Could you check a few things on this model? Use its own coordinates, in mm. Face numbers are marked on the shaded views. Round coordinates to 2 decimals unless told otherwise and drop trailing zeros. Write each loop counter-clockwise with the first axis right and the second up, starting at its lowest first coordinate (ties: lowest second). Pieces come first, ordered by that corner, then holes. Notation, with made-up numbers: (58.5, 80.25) -> (93.5, 80.25) arc R9 ccw to (93.5, 85.25) -> close; hole circle Ø8 at (6.25, 62.25). An arc over 180 degrees is marked (long way). Answer in a Markdown table with one row per item.
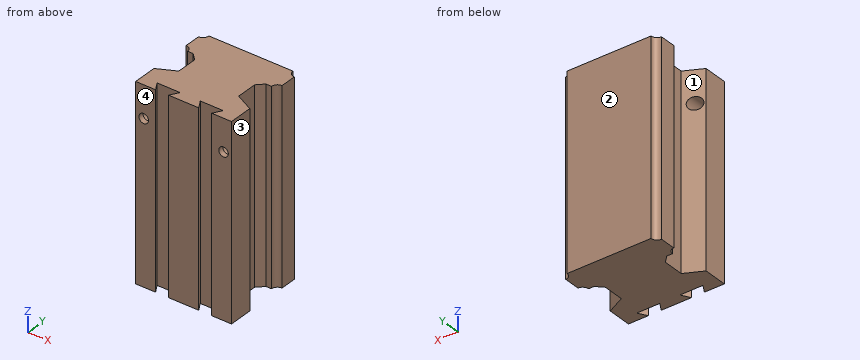
from build123d import *

# Parameters (mm, degrees)
BOSS_EXTRU_1_DEPTH        = 38.1
CONG_1_R                  = 2.38125
CHANFREIN1_SIZE           = 10.16
CHANFREIN1_SIZE_2         = 5.08
CHANFREIN2_SIZE           = 10.16
CHANFREIN2_SIZE_2         = 5.08
CHANFREIN3_SIZE           = 2.54
EMPREINTE1_START          = -38.1
EMPREINTE1_DEPTH          = 76.2
D_PLACER_START            = -38.1
D_PLACER_LA_FACE1_DEPTH   = 76.2
ESQUISSE4_W               = 1.89865
ESQUISSE4_H               = 21.2725
D_GAGEMENT_61_AT_2_COUNT  = 2
D_GAGEMENT_61_AT_2_PITCH  = 31.75
D_GAGEMENT_101_AT_2_COUNT = 2
D_GAGEMENT_101_AT_2_PITCH = 31.75


# Read off the part's stored shape, not the designer's step: Empreinte1, Déplacer la face1
# Some blends are built 0.0001 mm under size
with BuildPart() as part:
    # Esquisse2 → Boss.-Extru.1 (new, symmetric)
    with BuildSketch(Plane.XY):
        Polygon((-19.05, -15.875), (19.05, -15.875), (19.05, -7.9375), (11.90625, -7.9375), (11.90625, 7.9375), (16.66875, 7.9375), (16.66875, 10.31875), (19.05, 10.31875), (19.05, 16.66875), (16.66875, 16.66875), (16.66875, 19.05), (-16.66875, 19.05), (-16.66875, 16.66875), (-19.05, 16.66875), (-19.05, 10.31875), (-16.66875, 10.31875), (-16.66875, 7.9375), (-11.90625, 7.9375), (-11.90625, -7.9375), (-19.05, -7.9375), align=None)
    extrude(amount=BOSS_EXTRU_1_DEPTH, both=True)

    # Congé1
    cong_1_edges = [part.edges().sort_by_distance(p)[0] for p in [
        (-16.66875, 16.66875, 0),
        (-16.66875, 10.31875, 0),
        (16.66875, 10.31875, 0),
        (16.66875, 16.66875, 0),
    ]]
    fillet(cong_1_edges, radius=CONG_1_R - 0.0001)  # a hair under: the kernel refuses the full size

    # Chanfrein1
    # the kernel refuses this chamfer: 10.16, 5.08 mm, written as the material it adds along each edge
    with BuildSketch(Plane(origin=(-11.90625, -7.9375, 38.1), x_dir=(-0.9998508956747119, -0.017268075123668056, 0), z_dir=(0, 0, -1))) as chanfrein1_piece_1_section:
        Polygon((CHANFREIN1_SIZE * 0.999850895675, CHANFREIN1_SIZE * 0.0172680751237), (-CHANFREIN1_SIZE_2 * 0.0172680751237, CHANFREIN1_SIZE_2 * 0.999850895675), (0, 0), align=None)
    chanfrein1_piece_1 = extrude(amount=76.2, mode=Mode.PRIVATE)
    chanfrein1_piece_1 = split(chanfrein1_piece_1, bisect_by=Plane(origin=(-19.05, -6.161924143, 0), z_dir=(1, 0, 0)), keep=Keep.TOP, mode=Mode.PRIVATE)
    add(chanfrein1_piece_1)

    # Chanfrein2
    # the kernel refuses this chamfer: 10.16, 5.08 mm, written as the material it adds along each edge
    with BuildSketch(Plane(origin=(11.90625, -7.9375, -38.1), x_dir=(0.9998508956747119, -0.017268075123668056, 0), z_dir=(0, 0, 1))) as chanfrein2_piece_1_section:
        Polygon((CHANFREIN2_SIZE * 0.999850895675, CHANFREIN2_SIZE * 0.0172680751237), (-CHANFREIN2_SIZE_2 * 0.0172680751237, CHANFREIN2_SIZE_2 * 0.999850895675), (0, 0), align=None)
    chanfrein2_piece_1 = extrude(amount=76.2, mode=Mode.PRIVATE)
    chanfrein2_piece_1 = split(chanfrein2_piece_1, bisect_by=Plane(origin=(19.05, -6.161924143, 0), z_dir=(-1, 0, 0)), keep=Keep.TOP, mode=Mode.PRIVATE)
    add(chanfrein2_piece_1)

    # Chanfrein3
    chanfrein3_edges = [part.edges().sort_by_distance(p)[0] for p in [
        (-11.90625, 7.9375, 0),
        (11.90625, 7.9375, 0),
    ]]
    chamfer(chanfrein3_edges, length=CHANFREIN3_SIZE)

    # Empreinte1 outline → Empreinte1 (cut)
    with BuildSketch(Plane.XY.offset(EMPREINTE1_START)):
        Polygon((-6.278087105, -15.875), (-4.445, -12.7), (-12.7, -12.7), (-10.866912895, -15.875), align=None)
        Polygon((4.445, -12.7), (6.278087105, -15.875), (10.866912895, -15.875), (12.7, -12.7), align=None)
    extrude(amount=EMPREINTE1_DEPTH, mode=Mode.SUBTRACT)

    # Déplacer la face1 outline → Déplacer la face1 (cut)
    with BuildSketch(Plane.XY.offset(D_PLACER_START)):
        Polygon((-5.984793168, -15.875), (-4.005059095, -12.446), (-13.139940905, -12.446), (-11.160206832, -15.875), (-10.866912895, -15.875), (-12.7, -12.7), (-4.445, -12.7), (-6.278087105, -15.875), align=None)
        Polygon((4.005059095, -12.446), (5.984793168, -15.875), (6.278087105, -15.875), (4.445, -12.7), (12.7, -12.7), (10.866912895, -15.875), (11.160206832, -15.875), (13.139940905, -12.446), align=None)
    extrude(amount=D_PLACER_LA_FACE1_DEPTH, mode=Mode.SUBTRACT)

    # Esquisse4 → Dégagement #61 (revolve, cut)
    with BuildSketch(Plane(origin=(-15.875, 5.3975, 25.4), x_dir=(0, 0, 1), z_dir=(1, 0, 0))):
        with Locations((0.949325, 10.63625)):
            Rectangle(ESQUISSE4_W, ESQUISSE4_H)
    d_gagement_61 = revolve(axis=Axis((-15.875, 11.7475, 25.4), (0, -1, 0)), mode=Mode.SUBTRACT)

    # Dégagement #61 at 2: Dégagement #61 ×2
    with Locations(*[(i * D_GAGEMENT_61_AT_2_PITCH, 0, 0) for i in range(1, D_GAGEMENT_61_AT_2_COUNT)]):
        add(d_gagement_61, mode=Mode.SUBTRACT)

    # Esquisse7 → Dégagement #101 (revolve, cut)
    with BuildSketch(Plane(origin=(-15.875, 5.3975, 25.4), x_dir=(0, 0, 1), z_dir=(1, 0, 0))):
        Polygon((0, 0), (0, 20.329816902), (2.5527, 18.796), (2.5527, 0), align=None)
    d_gagement_101 = revolve(axis=Axis((-15.875, 11.7475, 25.4), (0, -1, 0)), mode=Mode.SUBTRACT)

    # Dégagement #101 at 2: Dégagement #101 ×2
    with Locations(*[(i * D_GAGEMENT_101_AT_2_PITCH, 0, 0) for i in range(1, D_GAGEMENT_101_AT_2_COUNT)]):
        add(d_gagement_101, mode=Mode.SUBTRACT)


solid = part.part
1) Imagine slicing it at D-D, the plane x = -7. Please give me the cut outline in (y, z).
Findings:
| item | result |
|---|---|
| outline | (-12.45, -38.1) -> (19.05, -38.1) -> (19.05, 38.1) -> (-12.45, 38.1) -> close |
2) Imagine slicing it at B-B, the plane y = 0. Please give me the cut outline in (x, z), plus the area to 3 significant figures.
Findings:
| item | result |
|---|---|
| outline | (-11.91, -38.1) -> (11.91, -38.1) -> (11.91, 38.1) -> (-11.91, 38.1) -> close |
| area | 1,810 mm^2 |
3) Imagine slicing it at A-A, the plane x = 5. Please give me the cut outline in (y, z) (3 decimals), plus the area to 3 significant figures.
Findings:
| item | result |
|---|---|
| outline | (-15.875, -38.1) -> (-14.169, -38.1) -> (-14.169, 38.1) -> (-15.875, 38.1) -> close; (-12.446, -38.1) -> (19.05, -38.1) -> (19.05, 38.1) -> (-12.446, 38.1) -> close |
| area | 2,530 mm^2 |
4) Imagine slicing it at C-C, the plane z = 25.4. Count the separate pieces of the cut face and the enclosed holes in it, plus the area to 3 significant figures.
Findings:
| item | result |
|---|---|
| separate pieces | 3 |
| enclosed holes | 0 |
| area | 984 mm^2 |
5) Please list where these lines run through material, in increasing order: line 1 (X direction, y = -14, z = 25); line 2 (Z direction, x = -16, y = -14); line 3 (Y direction, x = 12, z = 33) (3 decimals).
Findings:
| item | result |
|---|---|
| line 1 | x = -19.05 to -17.73, -14.02 to -12.24, -4.9 to 4.9, 12.24 to 14.02, 17.73 to 19.05 |
| line 2 | z = -38.1 to 23.51, 27.29 to 38.1 |
| line 3 | y = -15.875 to -14.42, -12.446 to -2.904, 5.491 to 19.05 |
6) Thinking about a two-plate mould opening in Y: for the marked faces 1, 2, 3 and 4, which applies, +Y half, -Y half, draft (parallel to the pull), parting line (faces both ways), or undercut?
Findings:
| item | result |
|---|---|
| face 1 | undercut |
| face 2 | +Y half |
| face 3 | draft |
| face 4 | -Y half |
7) For pin 1 (4 mm diameter, centred on y = 3, z = 5.5, fed in from +X); pin 2 (6 mm diameter, centred on y = 8.5, z = 11.5, fed in from +X); pin 3 (6 mm diameter, centred on y = -2.5, z = -16, fed in from -X); pin 4 (2.5 mm diameter, centred on y = 2.5, z = 2.5, fed in from -X), each with a flat end and sliding along its axis, tell me the tip position at first contact or that it passes through.
Findings:
| item | result |
|---|---|
| pin 1 | stops at x = 11.91 |
| pin 2 | stops at x = 19.05 |
| pin 3 | stops at x = -17.19 |
| pin 4 | stops at x = -11.91 |
